Source: CAD feature listing. Evaluate the final solid. Frame: model axes, mm. Face numbers are marked on the shaded views. A direction names the side the tool comes from. Round coordinates to 2 decimals unless told otherwise and drop trailing zeros. Order: outer loops, then holes, each group sorted by start corner. A loop starts at its lowest first (then second) coordinate and runs counter-clockwise, first axis right, second up. Notation, with made-up numbers: (31, -5.75) - (47, -5.75) arc R38 ccw to (47, 33.25) - close; hole circle Ø11 at (63.5, 2.25). An arc over 180 degrees is marked (long way). Put each result on its own line as item: value. Start each with the question number.
1) Mould query, pull axis Y, two halves, no side actions, for the marked faces 1, 2 and 3. Classes: +Y half, -Y half, draft (parallel to the pull), parting line (faces both ways), or undercut.
2) Section B-B on y = -4.5. Output: boundary loops of the cut face in (x, z), then the cut area to 4 significant figures.
3) Contact query for flat-ended pins moving along their axis: P1, Ø5, axis at x = -7.5, z = -27, coming from the +Y side; P2, Ø8, axis at x = -8.5, y = 0, coming from the -Z side; P3, Ø6, axis at x = 1.5, z = -19.5, coming from the -Y side. Output: stop coordinate, or through.
4) Access query for the marked faces 4, 5 and 6. Directions: +Z, -Z, +X, -X, +Y, -Y. A direction counts if a zero-diameter tool reaches every point of the face in a straight line with its end or side. Return the directions, or none.
5) Section D-D on z = -27. State how many separate pieces and enclosed holes the cut face has, then the cut area to 3 significant figures.
6) Line query: probe 1 along Y at (x, z) = (6, -20); probe 2 along X at (y, z) = (21.1, -27); probe 3 along Y at (x, z) = (-8.5, -9). Output: solid intervals per line, ascending. Write a range as [from, to].
7) Section A-A on z = -20.5. Output: boundary loops of the cut face in (x, y), then the cut area to 3 significant figures.
8) Section C-C on x = 2.25. Output: boundary loops of the cut face in (y, z).
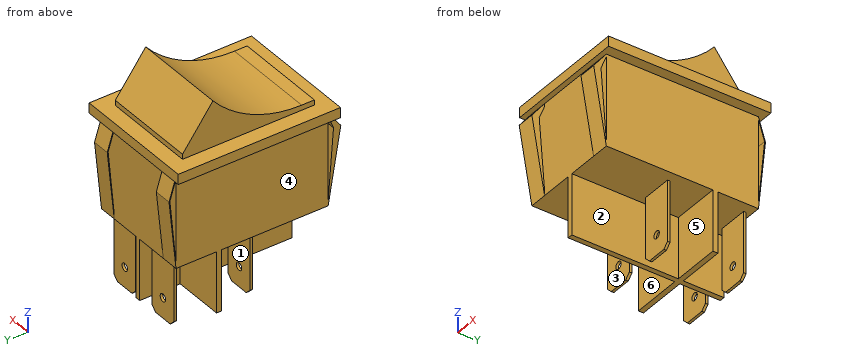
```python
from build123d import *

# Parameters (mm, degrees)
SKETCH1_W                = 24.5
SKETCH1_H                = 32
EXTRUDE2_DEPTH           = 2
SKETCH2_W                = 20.5
SKETCH2_H                = 30
EXTRUDE3_DEPTH           = 18
SKETCH4_W                = 18.5
SKETCH4_H                = 26
EXTRUDE7_DEPTH           = 1
EXTRUDE8_DEPTH           = 18.5
EXTRUDE9_DEPTH           = 3.5
EXTRUDE10_DEPTH          = 3.5
EXTRUDE11_DEPTH          = 3.5
EXTRUDE12_DEPTH          = 3.5
SKETCH10_W               = 1
SKETCH10_H               = 30
EXTRUDE13_DEPTH          = 12
SKETCH11_W               = 9.5
SKETCH11_H               = 1
SKETCH11_W_2             = 10
EXTRUDE14_DEPTH          = 12
SKETCH12_W               = 6
SKETCH12_H               = 0.5
EXTRUDE15_DEPTH          = 13
CHAMFER1_SIZE            = 1
SKETCH14_R               = 0.75
CUT_EXTRUDE2_DEPTH       = 1
TAGLIO_ESTRUSIONE1_REACH = 18.5
SKETCH13_R               = 0.75


with BuildPart() as part:
    # Sketch1 → Extrude2 (new body)
    with BuildSketch(Plane.XY):
        with Locations((-1.666405536, 7.433431257)):
            Rectangle(SKETCH1_W, SKETCH1_H)
    extrude(amount=EXTRUDE2_DEPTH)

    # Sketch2 → Extrude3 (add)
    with BuildSketch(Plane(origin=(0, 0, 0), x_dir=(-1, 0, 0), z_dir=(0, 0, -1))):
        with Locations((1.666405536, 7.433431257)):
            Rectangle(SKETCH2_W, SKETCH2_H)
    extrude(amount=EXTRUDE3_DEPTH)

    # Sketch4 → Extrude7 (add)
    with BuildSketch(Plane.XY.offset(2)):
        with Locations((-1.666405536, 7.433431257)):
            Rectangle(SKETCH4_W, SKETCH4_H)
    extrude(amount=EXTRUDE7_DEPTH)

    # Sketch5 → Extrude8 (add)
    with BuildSketch(Plane.ZY.offset(10.916405536)):
        with BuildLine():
            Line((3, 20.433431257), (3, -3.065691745))
            ThreePointArc((3, -3.065691745), (5.094825857, 6.554850155), (11, 14.433431257))
            Line((11, 14.433431257), (3, 20.433431257))
        make_face()
    extrude(amount=-EXTRUDE8_DEPTH)

    # Sketch6 → Extrude9 (add)
    with BuildSketch(Plane.ZY.offset(11.916405536)):
        Polygon((-18, 22.433431257), (-17, 22.433431257), (-4.359704833, 23.632529834), (-0.5, 22.433431257), (0, 22.433431257), (-4.430049233, 23.809719331), align=None)
    extrude(amount=-EXTRUDE9_DEPTH)

    # Sketch7 → Extrude10 (add)
    with BuildSketch(Plane(origin=(8.583594464, 0, 0), x_dir=(0, 0, -1), z_dir=(1, 0, 0))):
        Polygon((18, 22.433431257), (17.001667285, 22.433431257), (4.359704833, 23.632529834), (0.5, 22.433431257), (0, 22.433431257), (4.430049233, 23.809719331), align=None)
    extrude(amount=-EXTRUDE10_DEPTH)

    # Sketch8 → Extrude11 (add)
    with BuildSketch(Plane(origin=(8.583594464, 0, 0), x_dir=(0, 0, -1), z_dir=(1, 0, 0))):
        Polygon((0, -7.566568743), (0.5, -7.566568743), (3.14109092, -8.623937135), (17, -7.566568743), (18, -7.566568743), (3.237476094, -10.066568743), align=None)
    extrude(amount=-EXTRUDE11_DEPTH)

    # Sketch9 → Extrude12 (add)
    with BuildSketch(Plane.ZY.offset(11.916405536)):
        Polygon((0, -7.566568743), (-0.56008941, -7.566568743), (-3.14109092, -8.623937135), (-17, -7.566568743), (-18, -7.566568743), (-3.237476094, -10.066568743), align=None)
    extrude(amount=-EXTRUDE12_DEPTH)

    # Sketch10 → Extrude13 (add)
    with BuildSketch(Plane(origin=(0, 0, -18), x_dir=(-1, 0, 0), z_dir=(0, 0, -1))):
        with Locations((1.416405536, 7.433431257)):
            Rectangle(SKETCH10_W, SKETCH10_H)
    extrude(amount=EXTRUDE13_DEPTH)

    # Sketch11 → Extrude14 (add)
    with BuildSketch(Plane(origin=(0, 0, -18), x_dir=(-1, 0, 0), z_dir=(0, 0, -1))):
        with Locations((-3.833594464, 13.933431257)):
            Rectangle(SKETCH11_W, SKETCH11_H)
        with Locations((6.916405536, 13.933431257)):
            Rectangle(SKETCH11_W_2, SKETCH11_H)
    extrude(amount=EXTRUDE14_DEPTH)

    # Sketch12 → Extrude15 (add)
    with BuildSketch(Plane(origin=(0, 0, -18), x_dir=(-1, 0, 0), z_dir=(0, 0, -1))):
        with Locations((-3.583594464, 21.183431257)):
            Rectangle(SKETCH12_W, SKETCH12_H)
        with Locations((6.916405536, 21.183431257)):
            Rectangle(SKETCH12_W, SKETCH12_H)
        with Locations((-3.583594464, 6.183431257)):
            Rectangle(SKETCH12_W, SKETCH12_H)
        with Locations((6.916405536, 6.183431257)):
            Rectangle(SKETCH12_W, SKETCH12_H)
    extrude(amount=EXTRUDE15_DEPTH)

    # Chamfer1
    chamfer1_edges = [part.edges().sort_by_distance(p)[0] for p in [
        (6.583594464, 21.183431257, -31),
        (0.583594464, 21.183431257, -31),
        (-3.916405536, 21.183431257, -31),
        (-9.916405536, 21.183431257, -31),
        (6.583594464, 6.183431257, -31),
        (0.583594464, 6.183431257, -31),
        (-3.916405536, 6.183431257, -31),
        (-9.916405536, 6.183431257, -31),
    ]]
    chamfer(chamfer1_edges, length=CHAMFER1_SIZE)

    # Sketch14 → Cut-Extrude2 (cut)
    with BuildSketch(Plane(origin=(0, 21.433431257, 0), x_dir=(1, 0, 0), z_dir=(0, 1, 0))):
        with Locations((-6.916405536, 27)):
            Circle(SKETCH14_R)
        with Locations((3.583594464, 27)):
            Circle(SKETCH14_R)
    extrude(amount=-CUT_EXTRUDE2_DEPTH, mode=Mode.SUBTRACT)

    # Sketch13 → Taglio-Estrusione1 (cut, up to next)
    with BuildSketch(Plane.XZ.offset(-6.433431257), mode=Mode.PRIVATE) as taglio_estrusione1_sk1:
        with Locations((-6.916405536, -27)):
            Circle(SKETCH13_R)
    taglio_estrusione1_tool1 = extrude(taglio_estrusione1_sk1.sketch, amount=TAGLIO_ESTRUSIONE1_REACH, mode=Mode.PRIVATE) & part.part
    add(taglio_estrusione1_tool1.solids().sort_by_distance((-6.916406, 6.433431, -27))[0], mode=Mode.SUBTRACT)
    # Sketch13 → Taglio-Estrusione1 (cut, up to next)
    with BuildSketch(Plane.XZ.offset(-6.433431257), mode=Mode.PRIVATE) as taglio_estrusione1_sk2:
        with Locations((3.583594464, -27)):
            Circle(SKETCH13_R)
    taglio_estrusione1_tool2 = extrude(taglio_estrusione1_sk2.sketch, amount=TAGLIO_ESTRUSIONE1_REACH, mode=Mode.PRIVATE) & part.part
    add(taglio_estrusione1_tool2.solids().sort_by_distance((3.583594, 6.433431, -27))[0], mode=Mode.SUBTRACT)


solid = part.part
```
Answer sheet:
1. face 1: undercut
1. face 2: draft
1. face 3: -Y half
2. outline: (-13.92, 0) - (-11.92, 0) - (-11.92, -18) - (-1.92, -18) - (-1.92, -30) - (-0.92, -30) - (-0.92, -18) - (8.58, -18) - (8.58, 0) - (10.58, 0) - (10.58, 2) - (7.58, 2) - (7.58, 3) - (-10.92, 3) - (-10.92, 2) - (-13.92, 2) - close
2. area: 448.5 mm^2
3. P1: y = 21.43
3. P2: z = -18
3. P3: y = -7.57
4. face 4: -Z, -X, +Y, -Y
4. face 5: -Z, +X
4. face 6: -Z, -X
5. separate pieces: 9
5. enclosed holes: 0
5. area: 58.5 mm^2
6. probe 1: [5.93, 6.43], [13.43, 14.43], [20.93, 21.43]
6. probe 2: [-9.92, -7.67], [-6.17, -3.92], [-1.92, -0.92], [0.58, 2.83], [4.33, 6.58]
6. probe 3: [-9.09, -8.18], [-7.57, 22.43], [23.19, 23.35]
7. outline: (-11.92, 13.43) - (-1.92, 13.43) - (-1.92, -7.57) - (-0.92, -7.57) - (-0.92, 13.43) - (8.58, 13.43) - (8.58, 14.43) - (-0.92, 14.43) - (-0.92, 22.43) - (-1.92, 22.43) - (-1.92, 14.43) - (-11.92, 14.43) - close; (-9.92, 5.93) - (-3.92, 5.93) - (-3.92, 6.43) - (-9.92, 6.43) - close; (-9.92, 20.93) - (-3.92, 20.93) - (-3.92, 21.43) - (-9.92, 21.43) - close; (0.58, 5.93) - (6.58, 5.93) - (6.58, 6.43) - (0.58, 6.43) - close; (0.58, 20.93) - (6.58, 20.93) - (6.58, 21.43) - (0.58, 21.43) - close
7. area: 61.5 mm^2
8. outline: (-8.57, 0) - (-7.57, 0) - (-7.57, -18) - (5.93, -18) - (5.93, -31) - (6.43, -31) - (6.43, -18) - (13.43, -18) - (13.43, -30) - (14.43, -30) - (14.43, -18) - (20.93, -18) - (20.93, -31) - (21.43, -31) - (21.43, -18) - (22.43, -18) - (22.43, 0) - (23.43, 0) - (23.43, 2) - (20.43, 2) - (20.43, 3) - (14.43, 11) arc R23.14 cw to (-3.07, 3) - (-5.57, 3) - (-5.57, 2) - (-8.57, 2) - close
